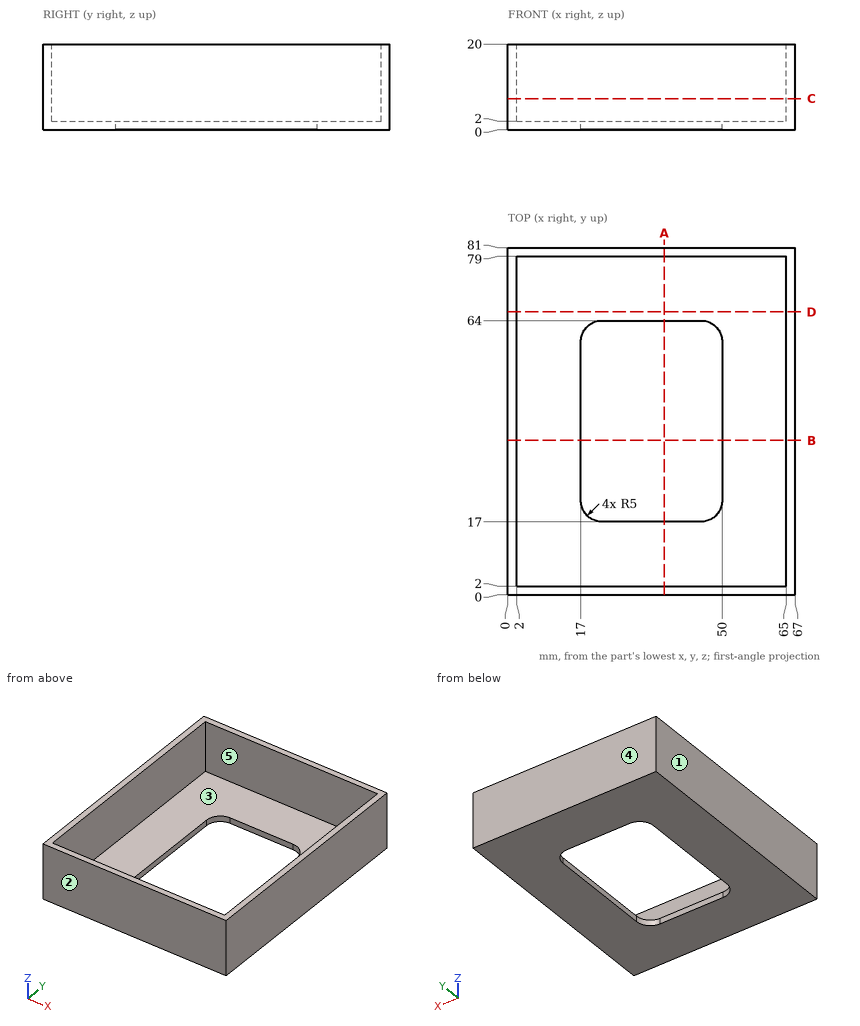
Here's the drawing with two shaded views (mm, measured from the low corner). I have some questions. A direction names the side the tool comes from. Give positions to 0.01 mm unless a question says otherwise; leave off trailing zeros. Loops run counter-clockwise (first coordinate to the right, second up) from the corner with the lowest first, then second, coordinate; pieces in that order, holes last. Notation, with made-up numbers: (73.25, 45) -> (86.25, 45) arc R19 ccw to (86.25, 70) -> close; hole circle Ø2 at (2.25, -8). An arc over 180 degrees is marked (long way). One line per item, written item: value.
Q1. If I drill on line 1 along Y through (x, z) = (10.5, 17.5); line 2 along X through (y, z) = (45, 9); line 3 along Z through (x, y) = (48, 13.5), over which ranges is the centre line in solid material (lowest first)?
Answers follow:
line 1: 0 to 2, 79 to 81
line 2: 0 to 2, 65 to 67
line 3: 0 to 2
Q2. I'm going to push a flat-ended pin straight in: pin 1 Ø6 at (x, y) = (10.5, 19) entering from +Z. Where does the tip first touch, or does it pass through?
Answers follow:
pin 1: z = 2
Q3. Suppose I cut it at A-A on x = 36.5. Please give me the cut outline in (y, z).
Answers follow:
outline: (0, 0) -> (17, 0) -> (17, 2) -> (2, 2) -> (2, 20) -> (0, 20) -> close; (64, 0) -> (81, 0) -> (81, 20) -> (79, 20) -> (79, 2) -> (64, 2) -> close
Q4. We'd pull the mould along X, two halves only. Please class the marked faces 1, 2 and 3: pulls with the +X half, pulls with the -X half, needs draft (parallel to the pull), parting line crosses it, or undercut.
Answers follow:
face 1: pulls with the -X half
face 2: needs draft
face 3: undercut
Q5. Suppose I cut it at C-C on z = 7.25. Please give me the cut outline in (x, y), then the cut area to 3 significant figures.
Answers follow:
outline: (0, 0) -> (67, 0) -> (67, 81) -> (0, 81) -> close; hole (2, 2) -> (65, 2) -> (65, 79) -> (2, 79) -> close
area: 576 mm^2
Q6. Suppose I cut it at D-D on y = 66. Please give me the cut outline in (x, z).
Answers follow:
outline: (0, 0) -> (67, 0) -> (67, 20) -> (65, 20) -> (65, 2) -> (2, 2) -> (2, 20) -> (0, 20) -> close
Q7. On a 3-axis mill with a long thin cutter (end or side, diameter ignored), from which of +Z, -Z, +X, -X, +Y, -Y can I reach the whole of each face in a straight line? I mean the marked faces 4 and 5. Say none if no direction works.
Answers follow:
face 4: +Z, -Z, +X, -X, +Y
face 5: +Z
Q8. Suppose I cut it at B-B on y = 36. Please give me the cut outline in (x, z).
Answers follow:
outline: (0, 0) -> (17, 0) -> (17, 2) -> (2, 2) -> (2, 20) -> (0, 20) -> close; (50, 0) -> (67, 0) -> (67, 20) -> (65, 20) -> (65, 2) -> (50, 2) -> close
